Source: CAD feature listing. Evaluate the final solid. Frame: model axes, mm. A direction names the side the tool comes from. Give positions to 0.01 mm unless a question says otherwise; leave off trailing zeros. Order: outer loops, then holes, each group sorted by start corner. A loop starts at its lowest first (then second) coordinate and runs counter-clockwise, first axis right, second up. Notation, with made-up numbers: M -34,-14.5 L 3,-14.5 A3 cw 3,-9.5 Z; hole C 12.25,12.5 d11. An arc over 180 degrees is marked long. Answer as a JSON object with one key per item and string values. Group by question number.
1. Section query D-D (y = 38.5). Output: boundary loops of the cut face in (x, z), plus the area to 3 significant figures.
2. Section query B-B (x = -14.5). Output: boundary loops of the cut face in (y, z), plus the area to 3 significant figures.
3. Material intervals for L1, parallel to Z at x = -9, y = 0.5; L2, parallel to X at y = 11, z = -1.5; L3, parallel to X at y = -47, z = -53, sorted ascending. Write a range as [from, to].
4. Pull-direction query (Z, two-part tool) for faces 4 (the cylindrical face through (2.416, -1.283, 90.986)), 5 (the flat face through (2, 58.35, 0)), 6 (the cylindrical face through (-2.7, -0.1, 77.4)); classes: +Z half, -Z half, draft (parallel to the pull), parting line (faces both ways), or undercut.
5. Set-up query: faces 1 (the flat face through (2, -58.35, 0)), 2 (the cylindrical face through (2.416, 1.283, -90.986)), 3 (the flat face through (-3, 3.3, -42)). Return all of +Z, -Z, +X, -X, +Y, -Y with unobstructed straight access to the full face (end or side cutting, diameter ignored); none if empty.
6. Pin query (flat end, axial travel): P1, Ø4.5, axis at x = -3, z = -48.5, coming from the +Y side; P2, Ø7.5, axis at x = -0.5, z = 29, coming from the -Y side; P3, Ø17, axis at x = -6.5, z = 45.5, coming from the +Y side. Return the tip coordinate at first contact, or that it passes through.
7. Section query A-A (y = 0). Output: boundary loops of the cut face in (x, z), plus the area to 3 significant figures.
8. Section query C-C (z = -65.5). Output: boundary loops of the cut face in (x, y).
from build123d import *

# Parameters (mm, degrees)
BOSS_EXTRUDE1_DEPTH = 4.9
BOSS_EXTRUDE2_DEPTH = 35
CUT_EXTRUDE1_DEPTH  = 122.049617926
BOSS_EXTRUDE3_DEPTH = 40
SKETCH4_R           = 151.595087716
CUT_EXTRUDE2_DEPTH  = 211.164221503
CUT_EXTRUDE3_DEPTH  = 210.547521178


with BuildPart() as part:
    # Sketch1 → Boss-Extrude1 (new body)
    with BuildSketch(Plane(origin=(0, 0, 0), x_dir=(0, 0, -1), z_dir=(1, 0, 0))):
        with BuildLine():
            Line((-32.65, 58.35), (32.65, 58.35))
            ThreePointArc((32.65, 58.35), (91, 0), (32.65, -58.35))
            Line((32.65, -58.35), (-32.65, -58.35))
            ThreePointArc((-32.65, -58.35), (-91, 0), (-32.65, 58.35))
        make_face()
    extrude(amount=BOSS_EXTRUDE1_DEPTH)

    # Sketch3 → Boss-Extrude2 (add)
    with BuildSketch(Plane.ZY):
        with BuildLine():
            Line((-58, 65), (58, 65))
            ThreePointArc((58, 65), (94, 0), (58, -65))
            Line((58, -65), (-58, -65))
            ThreePointArc((-58, -65), (-94, 0), (-58, 65))
        make_face()
    extrude(amount=BOSS_EXTRUDE2_DEPTH)

    # Sketch2 → Cut-Extrude1 (cut, through all)
    with BuildSketch(Plane(origin=(4.9, 0, 0), x_dir=(0, 0, -1), z_dir=(1, 0, 0))):
        with BuildLine():
            Line((-10.95, -3.3), (-74.1, -3.3))
            ThreePointArc((-74.1, -3.3), (-77.4, 0), (-74.1, 3.3))
            Line((-74.1, 3.3), (-10.95, 3.3))
            ThreePointArc((-10.95, 3.3), (-7.65, 0), (-10.95, -3.3))
        make_face()
        with BuildLine():
            Line((10.95, 3.3), (74.1, 3.3))
            ThreePointArc((74.1, 3.3), (77.4, 0), (74.1, -3.3))
            Line((74.1, -3.3), (10.95, -3.3))
            ThreePointArc((10.95, -3.3), (7.65, 0), (10.95, 3.3))
        make_face()
    extrude(amount=-CUT_EXTRUDE1_DEPTH, mode=Mode.SUBTRACT)

    # Sketch5 → Boss-Extrude3 (add)
    with BuildSketch(Plane(origin=(0, -65, -58), x_dir=(0, 0, -1), z_dir=(1, 0, 0))):
        with BuildLine():
            Line((-116, 0), (0, 0))
            ThreePointArc((0, 0), (-58, -20), (-116, 0))
        make_face()
        with BuildLine():
            Line((-116, 130), (0, 130))
            ThreePointArc((0, 130), (-58, 150), (-116, 130))
        make_face()
    extrude(amount=-BOSS_EXTRUDE3_DEPTH)

    # Sketch4 → Cut-Extrude2 (cut, through all)
    with BuildSketch(Plane(origin=(0, 0, -94), x_dir=(-1, 0, 0), z_dir=(0, 0, -1))):
        with Locations((162.145087716, 0)):
            Circle(SKETCH4_R)
    extrude(amount=-CUT_EXTRUDE2_DEPTH, mode=Mode.SUBTRACT)

    # Sketch8 → Cut-Extrude3 (cut, through all)
    with BuildSketch(Plane(origin=(0, 0, -94), x_dir=(-1, 0, 0), z_dir=(0, 0, -1))):
        Polygon((0, 65), (0, 85), (20.321882247, 85), align=None)
        Polygon((0, -65), (0, -85), (20.321882247, -85), align=None)
    extrude(amount=-CUT_EXTRUDE3_DEPTH, mode=Mode.SUBTRACT)


solid = part.part
Answer sheet:
{
 "1": {"outline": "M -15.52,-83.63 L 0,-83.63 L 0,-76.5 L 4.9,-76.5 L 4.9,76.5 L 0,76.5 L 0,83.63 L -15.52,83.63 Z", "area": "3,350 mm^2"},
 "2": {"outline": "M -79.27,-32.33 A94.1 ccw -65,-58 A76.68 ccw -34.38,-85.86 L -34.38,85.86 A76.68 ccw -65,58 A94.1 ccw -79.27,32.33 Z; M 34.38,-85.86 A76.68 ccw 65,-58 A94.1 ccw 79.27,-32.33 L 79.27,32.33 A94.1 ccw 65,58 A76.68 ccw 34.38,85.86 Z", "area": "11,800 mm^2"},
 "3": {"L1": "[-94, -77.36], [-7.69, 7.69], [77.36, 94]", "L2": "[-10.95, 4.9]", "L3": "[-18.02, 4.9]"},
 "4": {"face 4": "+Z half", "face 5": "draft", "face 6": "undercut"},
 "5": {"face 1": "+Z, -Z, +X, -Y", "face 2": "-Z, +X", "face 3": "+X, -X"},
 "6": {"P1": "y = 70.17", "P2": "y = -69.18", "P3": "y = 76.61"},
 "7": {"outline": "M -10.55,-94 L 0,-94 L 0,-91 L 4.9,-91 L 4.9,-77.4 L -10.55,-77.4 Z; M -10.55,-7.65 L 4.9,-7.65 L 4.9,7.65 L -10.55,7.65 Z; M -10.55,77.4 L 4.9,77.4 L 4.9,91 L 0,91 L 0,94 L -10.55,94 Z", "area": "720 mm^2"},
 "8": {"outline": "M -22.78,-59.65 L 0,-59.65 L 0,-48.22 L 4.9,-48.22 L 4.9,-3.3 L -10.59,-3.3 A151.6 cw Z; M -22.78,59.65 A151.6 cw -10.59,3.3 L 4.9,3.3 L 4.9,48.22 L 0,48.22 L 0,59.65 Z"}
}
